Input: part model. Units: mm. Frame: model coordinates. A direction names the side the tool comes from. Give positions to 0.01 mm unless a question says otherwise; leave off trailing zeros. Write each loop counter-clockwise with the first axis right and the second up, starting at its lowest first coordinate (ties: lowest second). Pieces come first, ordered by that corner, then holes. Notation, with made-up numbers: M 62.25,-10 L 74.25,-10 A16 cw 74.25,2 Z; hole C 52,59 d5. An arc over 180 degrees is marked long. Use CSV: the item, a comma, the result in double quotes. Start each with the question number.
from build123d import *

# Parameters (mm, degrees)
SKETCH1_W                    = 70
SKETCH1_H                    = 70
BASE_FLANGE1_DEPTH           = 2
EDGE_FLANGE1_STRIP_W         = 9.4732
EDGE_FLANGE1_STRIP_H         = 2
EDGE_FLANGE1_STRIP_CUT_DEPTH = 70
EDGE_FLANGE1_DEPTH           = 70
SKETCH9_R                    = 8
CUT_EXTRUDE1_DEPTH           = 10
SKETCH11_R                   = 8
SKETCH11_R_2                 = 2
CUT_EXTRUDE2_DEPTH           = 10


# Sheet-metal steps are written as plain solids
with BuildPart() as part:
    # Sketch1 → Base-Flange1 (new body)
    with BuildSketch(Plane(origin=(0, 0, 0), x_dir=(1, 0, 0), z_dir=(0, 1, 0))):
        Rectangle(SKETCH1_W, SKETCH1_H)
    extrude(amount=-BASE_FLANGE1_DEPTH)

    # Edge-Flange1 strip (across the edge) → Edge-Flange1 strip cut (cut)
    with BuildSketch(Plane(origin=(35, 0, -35), x_dir=(0, 0, 1), z_dir=(-1, 0, 0))):
        with Locations((-4, -1)):
            Rectangle(EDGE_FLANGE1_STRIP_W, EDGE_FLANGE1_STRIP_H)
    extrude(amount=EDGE_FLANGE1_STRIP_CUT_DEPTH, mode=Mode.SUBTRACT)

    # Edge-Flange1 section (across the edge) → Edge-Flange1 (add)
    with BuildSketch(Plane(origin=(35, 0, -35), x_dir=(0, 0, 1), z_dir=(-1, 0, 0))):
        with BuildLine():
            Line((-2, 0.7366), (-2, 30))
            Line((-2, 30), (0, 30))
            Line((0, 30), (0, 0.7366))
            ThreePointArc((0, 0.7366), (0.215745145, 0.215745145), (0.7366, 0))
            Line((0.7366, 0), (0.7366, -2))
            ThreePointArc((0.7366, -2), (-1.198468417, -1.198468417), (-2, 0.7366))
        make_face()
    extrude(amount=EDGE_FLANGE1_DEPTH)

    # Sketch9 → Cut-Extrude1 (cut)
    with BuildSketch(Plane.XY.offset(-35)):
        with Locations((0, 15)):
            Circle(SKETCH9_R)
    extrude(amount=-CUT_EXTRUDE1_DEPTH, mode=Mode.SUBTRACT)

    # Sketch11 → Cut-Extrude2 (cut)
    with BuildSketch(Plane.XZ.offset(2)):
        with Locations(Location((0, 20, 0), (0, 0, 270))):
            Circle(SKETCH11_R)
        with Locations(Location((-27, 25, 0), (0, 0, 270))):
            Circle(SKETCH11_R_2)
        with Locations(Location((-19, 15, 0), (0, 0, 270))):
            Circle(SKETCH11_R_2)
        with Locations(Location((-27, 5, 0), (0, 0, 270))):
            Circle(SKETCH11_R_2)
        with Locations(Location((-19, -5, 0), (0, 0, 270))):
            Circle(SKETCH11_R_2)
        with Locations(Location((-27, -15, 0), (0, 0, 270))):
            Circle(SKETCH11_R_2)
        with Locations(Location((-19, -25, 0), (0, 0, 270))):
            Circle(SKETCH11_R_2)
        with Locations(Location((27, 5, 0), (0, 0, 90))):
            Circle(SKETCH11_R_2)
        with Locations(Location((19, 15, 0), (0, 0, 90))):
            Circle(SKETCH11_R_2)
        with Locations(Location((19, -25, 0), (0, 0, 90))):
            Circle(SKETCH11_R_2)
        with Locations(Location((27, -15, 0), (0, 0, 90))):
            Circle(SKETCH11_R_2)
        with Locations(Location((19, -5, 0), (0, 0, 90))):
            Circle(SKETCH11_R_2)
        with Locations(Location((27, 25, 0), (0, 0, 90))):
            Circle(SKETCH11_R_2)
    extrude(amount=-CUT_EXTRUDE2_DEPTH, mode=Mode.SUBTRACT)


solid = part.part
Q1. First-contact query: pin 1 Ø4.5 at (x, z) = (-27, 5) entering from +Y; pin 2 Ø3 at (x, z) = (27, -15) entering from +Y; pin 3 Ø9 at (x, y) = (-17, 14) entering from +Z. Flat tips, straight axial feed; report the tip coordinate or a pass-through.
Q2. Material intervals for L1, parallel to X at y = -0.55, z = -5; L2, parallel to X at y = -0.85, z = -15; L3, parallel to X at y = -1.1, z = 20, sorted ascending. Write a range as [from, to].
Q3. Section A-A, the plane z = -5. Return the cut outline in (x, y), and give its area (3 significant figures).
Q4. Set-up query: faces 5 (the cylindrical face through (-17, -1, 15)), 6 (the flat face through (8.3, 15.6, -35)). Return all of +Z, -Z, +X, -X, +Y, -Y with unobstructed straight access to the full face (end or side cutting, diameter ignored); none if empty.
Q5. Section C-C, the plane z = 20. Return the cut outline in (x, y).
Q6. Section B-B, the plane y = 15. Return the cut outline in (x, z), and give its area (3 significant figures).
Q7. Section D-D, the plane x = 0. Return the cut outline in (y, z), and give its area (3 significant figures).
Q8. Pull-direction query (Z, two-part tool) for faces 1 (the cylindrical face through (-4.868, -1.014, 26.349)), 2 (the cylindrical face through (0.49, -1.22, -36.177)), 3 (the cylindrical face through (-29, -1, 25)), 4 (the flat face through (35, -1, -11)); classes: released by +Z, released by -Z, zero draft, split by the parting line, or undercut.
Check result:
1,pin 1,"stops at y = 0"
1,pin 2,"passes through"
1,pin 3,"stops at z = -35"
2,L1,"x = [-35, -21], [-17, 17], [21, 35]"
2,L2,"x = [-35, -29], [-25, 25], [29, 35]"
2,L3,"x = [-35, -8], [8, 35]"
3,outline,"M -35,-2 L -21,-2 L -21,0 L -35,0 Z; M -17,-2 L 17,-2 L 17,0 L -17,0 Z; M 21,-2 L 35,-2 L 35,0 L 21,0 Z"
3,area,"124 mm²"
4,face 5,"+Y, -Y"
4,face 6,"+Z, +X, -X, +Y"
5,outline,"M -35,-2 L -8,-2 L -8,0 L -35,0 Z; M 8,-2 L 35,-2 L 35,0 L 8,0 Z"
6,outline,"M -35,-37 L -8,-37 L -8,-35 L -35,-35 Z; M 8,-37 L 35,-37 L 35,-35 L 8,-35 Z"
6,area,"108 mm²"
7,outline,"M -2,-34.26 A2.74 ccw 0.74,-37 L 7,-37 L 7,-35 L 0.74,-35 A0.74 cw 0,-34.26 L 0,12 L -2,12 Z; M -2,28 L 0,28 L 0,35 L -2,35 Z; M 23,-37 L 30,-37 L 30,-35 L 23,-35 Z"
7,area,"139 mm²"
8,face 1,"undercut"
8,face 2,"released by -Z"
8,face 3,"undercut"
8,face 4,"zero draft"
